Source: CAD feature listing. Evaluate the final solid. Frame: model axes, mm. A direction names the side the tool comes from. Give positions to 0.01 mm unless a question says otherwise; leave off trailing zeros. Order: outer loops, then holes, each group sorted by start corner. A loop starts at its lowest first (then second) coordinate and runs counter-clockwise, first axis right, second up. Notation, with made-up numbers: (32, 4) - (79, 4) arc R10 ccw to (79, 20) - close; hole circle Ø11 at (27.25, 87.5). An arc over 180 degrees is marked (long way). Answer as CSV lines item,"result".
```python
from build123d import *

# Parameters (mm, degrees)
SKETCH1_W      = 15
SKETCH1_H      = 25
EXTRUDE1_DEPTH = 5
SKETCH2_W      = 15
SKETCH2_H      = 5
EXTRUDE2_DEPTH = 10
SKETCH3_R      = 1.5
EXTRUDE3_DEPTH = 10
SKETCH4_R      = 1.5
EXTRUDE4_DEPTH = 10


with BuildPart() as part:
    # Sketch1 → Extrude1 (new body)
    with BuildSketch(Plane(origin=(0, 0, 0), x_dir=(1, 0, 0), z_dir=(0, 1, 0))):
        Rectangle(SKETCH1_W, SKETCH1_H)
    extrude(amount=EXTRUDE1_DEPTH)

    # Sketch2 → Extrude2 (add)
    with BuildSketch(Plane(origin=(0, 5, 0), x_dir=(1, 0, 0), z_dir=(0, 1, 0))):
        with Locations((0, 10)):
            Rectangle(SKETCH2_W, SKETCH2_H)
    extrude(amount=EXTRUDE2_DEPTH)

    # Sketch3 → Extrude3 (cut)
    with BuildSketch(Plane(origin=(0, 5, 0), x_dir=(1, 0, 0), z_dir=(0, 1, 0))):
        with Locations(Location((0, -7.5, 0), (0, 0, 270))):
            Circle(SKETCH3_R)
    extrude(amount=-EXTRUDE3_DEPTH, mode=Mode.SUBTRACT)

    # Sketch4 → Extrude4 (cut)
    with BuildSketch(Plane.XY.offset(-7.5)):
        with Locations((0, 10)):
            Circle(SKETCH4_R)
    extrude(amount=-EXTRUDE4_DEPTH, mode=Mode.SUBTRACT)


solid = part.part
```
(1) Cut plane B-B (y = 10). Return loops of the section in (x, z), then the cut area to 3 significant figures.
Completed:
outline,"(-7.5, -12.5) - (-1.5, -12.5) - (-1.5, -7.5) - (-7.5, -7.5) - close; (1.5, -12.5) - (7.5, -12.5) - (7.5, -7.5) - (1.5, -7.5) - close"
area,"60.0 mm²"
(2) Cut plane C-C (z = -10.25). Return loops of the section in (x, y).
Completed:
outline,"(-7.5, 0) - (7.5, 0) - (7.5, 15) - (-7.5, 15) - close; hole circle Ø3 at (0, 10)"
(3) Ray query, line 1 (Y direction, x = 0, z = -9.05); line 2 (X direction, y = 4, z = 7.5); line 3 (Z direction, x = -4.25, y = 9.5). Return the intervals inside material, ascending. Write a range as from..to.
Completed:
line 1,"0..8.5, 11.5..15"
line 2,"-7.5..-1.5, 1.5..7.5"
line 3,"-12.5..-7.5"
(4) Contact query for a flat-ended pin moving along its axis: pin 1 (3 mm diameter, centred on x = 3.5, y = 10.5, fed in from +Z). Output: stop coordinate, or through.
Completed:
pin 1,"z = -7.5"
(5) Access query for faces 4 (the flat face through (-2, 10, -7.5)), 5 (the cylindrical face through (0, 3, 6)). Directions: +Z, -Z, +X, -X, +Y, -Y. A direction counts if a zero-diameter tool reaches every point of the face in a straight line with its end or side. Return the directions, or none.
Completed:
face 4,"+Z, +X, -X, +Y"
face 5,"+Y, -Y"
(6) Cut plane D-D (z = 7.5). Return loops of the section in (x, y).
Completed:
outline,"(-7.5, 0) - (-1.5, 0) - (-1.5, 5) - (-7.5, 5) - close; (1.5, 0) - (7.5, 0) - (7.5, 5) - (1.5, 5) - close"
(7) Mould query, pull axis Y, two halves, no side actions, for faces 1 (the flat face through (0, 0, 0)), 2 (the cylindrical face through (-0.325, 8.536, -9.965)), 3 (the flat face through (7.5, 4, -3)). Classes: released by +Y, released by -Y, zero draft, split by the parting line, or undercut.
Completed:
face 1,"released by -Y"
face 2,"undercut"
face 3,"zero draft"
(8) Cut plane A-A (x = 0). Return loops of the section in (y, z), then the cut area to 3 significant figures.
Completed:
outline,"(0, -12.5) - (8.5, -12.5) - (8.5, -7.5) - (5, -7.5) - (5, 6) - (0, 6) - close; (0, 9) - (5, 9) - (5, 12.5) - (0, 12.5) - close; (11.5, -12.5) - (15, -12.5) - (15, -7.5) - (11.5, -7.5) - close"
area,"145 mm²"
